Check sheet for the drawn part. Datum: minimum x, y, z corner. Units: mm. Round coordinates to 2 decimals unless told otherwise and drop trailing zeros. Write each loop counter-clockwise with the first axis right and the second up, starting at its lowest first coordinate (ties: lowest second). Pieces come first, ordered by that corner, then holes. Notation, with made-up numbers: M 44,21.5 L 84,21.5 A21 ccw 84,48.5 Z; hole C -40,9 d6. An arc over 180 degrees is marked long. One line per item, written item: value. Start each with the question number.
1. Depth check by flat-ended pin: P1, Ø1.5, axis at x = 202, z = 7.5, coming from the +Y side; P2, Ø2.5, axis at y = 119, z = 8.5, coming from the -X side; P3, Ø0.9, axis at y = 1, z = 8, coming from the +X side. Enter the tip coordinate at first touch or a pass-through.
2. Section check A-A (z = 8.5). Record the boundary of the cut face in (x, y).
3. Section check C-C (y = 72). Record the boundary of the cut face in (x, z).
4. Section check D-D (x = 33). Record the boundary of the cut face in (y, z), and give its area (3 significant figures).
5. Scan lines: probe 1 along Z at (x, y) = (116, 50.5); probe 2 along X at (y, z) = (58, 8.5); probe 3 along Y at (x, z) = (30, 4). Record each from-to range of solid material in increasing order. Write a range as [from, to].
6. Section check B-B (x = 101.5). Record the boundary of the cut face in (y, z), and give its area (3 significant figures).
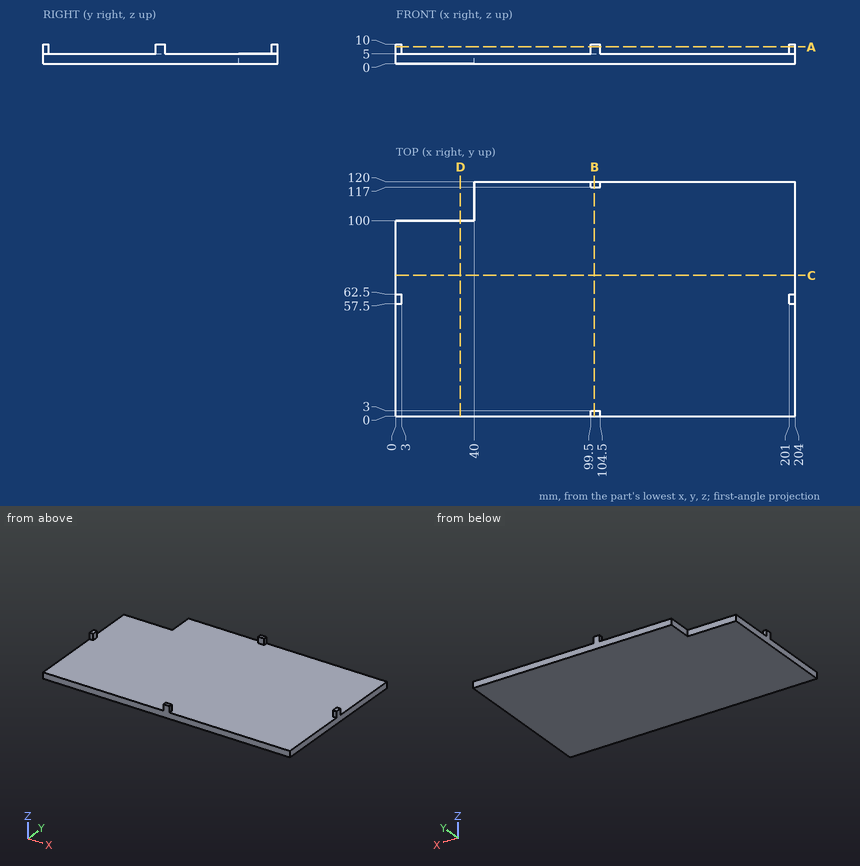
Result sheet:
1. P1: stops at y = 62.5
1. P2: stops at x = 99.5
1. P3: stops at x = 104.5
2. outline: M 0,57.5 L 3,57.5 L 3,62.5 L 0,62.5 Z; M 99.5,0 L 104.5,0 L 104.5,3 L 99.5,3 Z; M 99.5,117 L 104.5,117 L 104.5,120 L 99.5,120 Z; M 201,57.5 L 204,57.5 L 204,62.5 L 201,62.5 Z
3. outline: M 0,0 L 204,0 L 204,5 L 0,5 Z
4. outline: M 0,0 L 100,0 L 100,5 L 0,5 Z
4. area: 500 mm2
5. probe 1: z = [0, 5]
5. probe 2: x = [0, 3], [201, 204]
5. probe 3: y = [0, 100]
6. outline: M 0,0 L 120,0 L 120,10 L 117,10 L 117,5 L 3,5 L 3,10 L 0,10 Z
6. area: 630 mm2
